The drawing under review shows one solid part. Ordinate dimensions are in mm from its lowest x, y, z. Give positions to 0.01 mm unless a question says otherwise; leave off trailing zeros. Loops run counter-clockwise (first coordinate to the right, second up) from the corner with the lowest first, then second, coordinate; pieces in that order, holes last. Notation, with made-up numbers: M 81.5,45 L 95.5,45 A25 ccw 95.5,60 Z; hole C 29,-3.5 d11. An arc over 180 degrees is marked long. One line per item, written item: value. Start each with the question number.
Q1. We need section C-C on x = 3.5. Write out the cut boundary in (y, z) (3 decimals).
Q2. We need section D-D on z = 0.7. Give the number of separate pieces and of enclosed holes in the cut face, plus the area to 3 significant figures.
Q3. To check wall thickness, follow line 1 along Y through (x, z) = (40, 0.9); line 2 along X through (y, z) = (3.5, 0.75); line 3 along Y through (x, z) = (40.5, 0.7). State the ranges of each line that lie inside material, in increasing order. Write a range as from..to.
Q4. We need section B-B on y = 9. Write out the cut boundary in (x, z) (3 decimals), plus the area to 3 significant figures.
Q5. We need section A-A on x = 16. Write out the cut boundary in (y, z).
Q6. For pin 1 (3 mm diameter, centred on x = 44.5, y = 7, fed in from -Z); pin 2 (1 mm diameter, centred on x = 10, y = 10.27, fed in from -Z), all flat-tipped, find the tip position at first contact; note any pin that passes through.
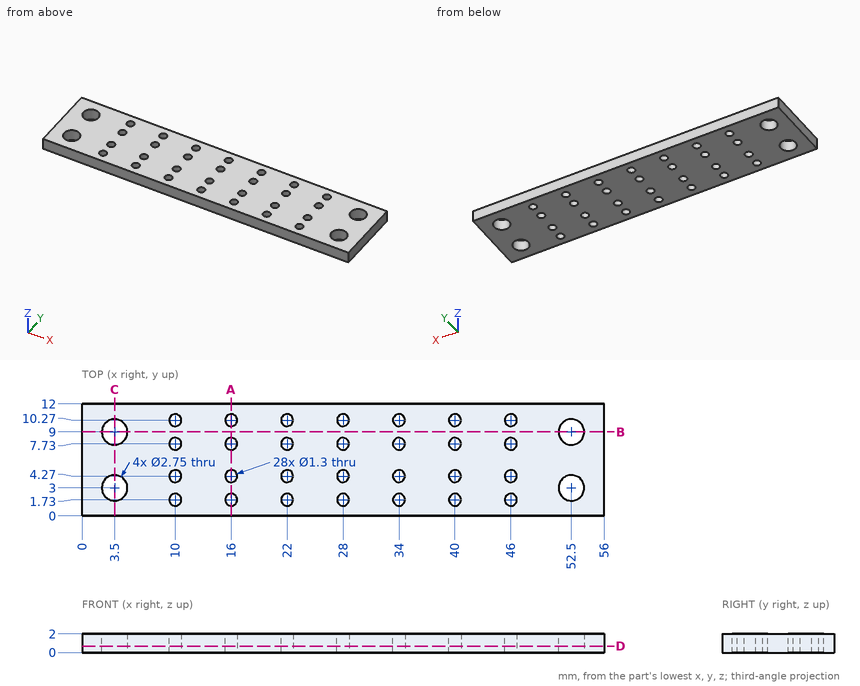
Solved:
1. outline: M 0,0 L 1.625,0 L 1.625,2 L 0,2 Z; M 4.375,0 L 7.625,0 L 7.625,2 L 4.375,2 Z; M 10.375,0 L 12,0 L 12,2 L 10.375,2 Z
2. separate pieces: 1
2. enclosed holes: 32
2. area: 611 mm2
3. line 1: 0..1.08, 2.38..3.62, 4.92..7.08, 8.38..9.62, 10.92..12
3. line 2: 0..2.22, 4.78..51.22, 53.78..56
3. line 3: 0..1.31, 2.15..3.85, 4.69..7.31, 8.15..9.85, 10.69..12
4. outline: M 0,0 L 2.125,0 L 2.125,2 L 0,2 Z; M 4.875,0 L 51.125,0 L 51.125,2 L 4.875,2 Z; M 53.875,0 L 56,0 L 56,2 L 53.875,2 Z
4. area: 101 mm2
5. outline: M 0,0 L 1.08,0 L 1.08,2 L 0,2 Z; M 2.38,0 L 3.62,0 L 3.62,2 L 2.38,2 Z; M 4.92,0 L 7.08,0 L 7.08,2 L 4.92,2 Z; M 8.38,0 L 9.62,0 L 9.62,2 L 8.38,2 Z; M 10.92,0 L 12,0 L 12,2 L 10.92,2 Z
6. pin 1: z = 0
6. pin 2: through
